The listing builds one solid part. Answer for the finished solid, in the listing's coordinates (mm). Round coordinates to 2 decimals unless told otherwise and drop trailing zeros. Loops run counter-clockwise (first coordinate to the right, second up) from the corner with the lowest first, then second, coordinate; pieces in that order, holes last. Notation, with made-up numbers: (80, -37) -> (89, -37) arc R22 cw to (89, -25) -> close; hole circle Ø3 at (-23.75, 5). An arc over 180 degrees is marked (long way). One line per question, with ' | ' between items.
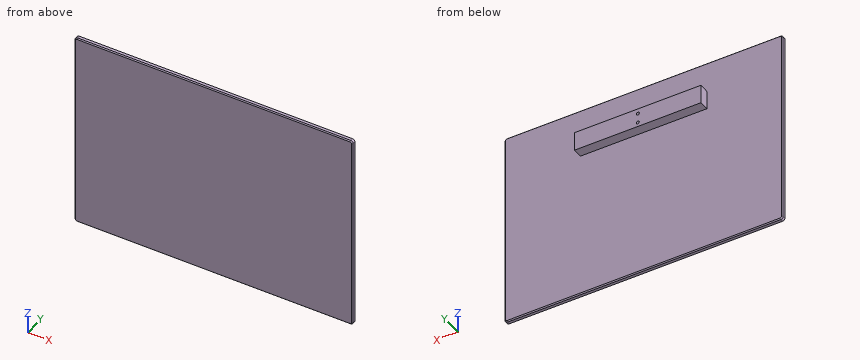
from build123d import *

# Parameters (mm, degrees)
SKETCH1_W           = 550
SKETCH1_H           = 400
BOSS_EXTRUDE1_DEPTH = 9.525
FILLET2_R           = 5
CHAMFER1_SIZE       = 2
CHAMFER2_SIZE       = 2
SKETCH3_W           = 250
SKETCH3_H           = 38.1
SKETCH3_R           = 3
BOSS_EXTRUDE2_DEPTH = 19.05


with BuildPart() as part:
    # Sketch1 → Boss-Extrude1 (new body)
    with BuildSketch(Plane(origin=(0, 0, 0), x_dir=(1, 0, 0), z_dir=(0, 1, 0))):
        Rectangle(SKETCH1_W, SKETCH1_H)
    extrude(amount=BOSS_EXTRUDE1_DEPTH)

    # Fillet2
    fillet2_edges = [part.edges().sort_by_distance(p)[0] for p in [
        (275, 4.7625, 200),
        (-275, 4.7625, 200),
        (-275, 4.7625, -200),
        (275, 4.7625, -200),
    ]]
    fillet(fillet2_edges, radius=FILLET2_R)

    # Chamfer1
    chamfer1_edges = [part.edges().sort_by_distance(p)[0] for p in [
        (-275, 9.525, 0),
        (0, 9.525, -200),
        (275, 9.525, 0),
        (0, 9.525, 200),
        (-273.535533906, 9.525, 198.535533906),
        (273.535533906, 9.525, 198.535533906),
        (273.535533906, 9.525, -198.535533906),
        (-273.535533906, 9.525, -198.535533906),
    ]]
    chamfer(chamfer1_edges, length=CHAMFER1_SIZE)

    # Chamfer2
    chamfer2_edges = [part.edges().sort_by_distance(p)[0] for p in [
        (-275, 0, 0),
        (275, 0, 0),
        (0, 0, 200),
        (0, 0, -200),
        (-273.535533906, 0, 198.535533906),
        (273.535533906, 0, 198.535533906),
        (273.535533906, 0, -198.535533906),
        (-273.535533906, 0, -198.535533906),
    ]]
    chamfer(chamfer2_edges, length=CHAMFER2_SIZE)

    # Sketch3 → Boss-Extrude2 (add)
    with BuildSketch(Plane(origin=(0, 9.525, 0), x_dir=(1, 0, 0), z_dir=(0, 1, 0))):
        with Locations((0, -119.4)):
            Rectangle(SKETCH3_W, SKETCH3_H)
        with Locations((0, -109.15)):
            Circle(SKETCH3_R, mode=Mode.SUBTRACT)
        with Locations((0, -128.25)):
            Circle(SKETCH3_R, mode=Mode.SUBTRACT)
    extrude(amount=BOSS_EXTRUDE2_DEPTH)


solid = part.part
Q1. A cutting plane is placed at B-B on x = -100.5. Give the vertices of the cut face in (y, z) (3 decimals), plus the area to 3 significant figures.
Numbers:
outline: (0, -198) -> (2, -200) -> (7.525, -200) -> (9.525, -198) -> (9.525, 100.35) -> (28.575, 100.35) -> (28.575, 138.45) -> (9.525, 138.45) -> (9.525, 198) -> (7.525, 200) -> (2, 200) -> (0, 198) -> close | area: 4,530 mm^2
Q2. Find the intervals of material crossed by line 1 (Z direction, x = 0, y = 16); line 2 (X direction, y = 19, z = 109.15); line 3 (Y direction, x = -203, z = -73.5) (3 decimals), in increasing order. Write a range as from..to.
Numbers:
line 1: 100.35..106.15, 112.15..125.25, 131.25..138.45 | line 2: -125..-3, 3..125 | line 3: 0..9.525
Q3. A cutting plane is placed at C-C on z = 153. Give the vertices of the cut face in (x, y) (3 decimals).
Numbers:
outline: (-275, 2) -> (-273, 0) -> (273, 0) -> (275, 2) -> (275, 7.525) -> (273, 9.525) -> (-273, 9.525) -> (-275, 7.525) -> close
Q4. A cutting plane is placed at D-D on x = 184.5. Give the vertices of the cut face in (y, z) (3 decimals).
Numbers:
outline: (0, -198) -> (2, -200) -> (7.525, -200) -> (9.525, -198) -> (9.525, 198) -> (7.525, 200) -> (2, 200) -> (0, 198) -> close
Q5. Given pin 1 Ø1.5 at (y, z) = (9.5, -94) entering from +X (3 decimals); pin 2 Ø2 at (x, z) = (72, 61) entering from +Y (3 decimals); pin 3 Ø5.5 at (x, y) = (-15.5, 18.5) entering from +Z, each flat-ended and moving along its own axis, determine where each tip first touches the part or whether it passes through.
Numbers:
pin 1: x = 273.775 | pin 2: y = 9.525 | pin 3: z = 138.45
Q6. A cutting plane is placed at A-A on y = 22.75. Give the vertices of the cut face in (x, z).
Numbers:
outline: (-125, 100.35) -> (125, 100.35) -> (125, 138.45) -> (-125, 138.45) -> close; hole circle Ø6 at (0, 109.15); hole circle Ø6 at (0, 128.25)
